Study the drawing (mm; zero at the part's minimum x, y, z) and answer. A direction names the side the tool comes from. Coordinates: 2 decimals unless noted, no trailing zeros. Write each loop counter-clockwise with the first axis right and the second up, starting at its lowest first coordinate (ties: lowest second). Pieces come first, ordered by that corner, then holes. Notation, with made-up numbers: M 55.25,-1.75 L 108.25,-1.75 A25 ccw 108.25,11.25 Z; hole C 55.5,74.25 d11. An arc over 180 degrees is marked long. Answer as a JSON object with one key per item and string values. Group by question number.
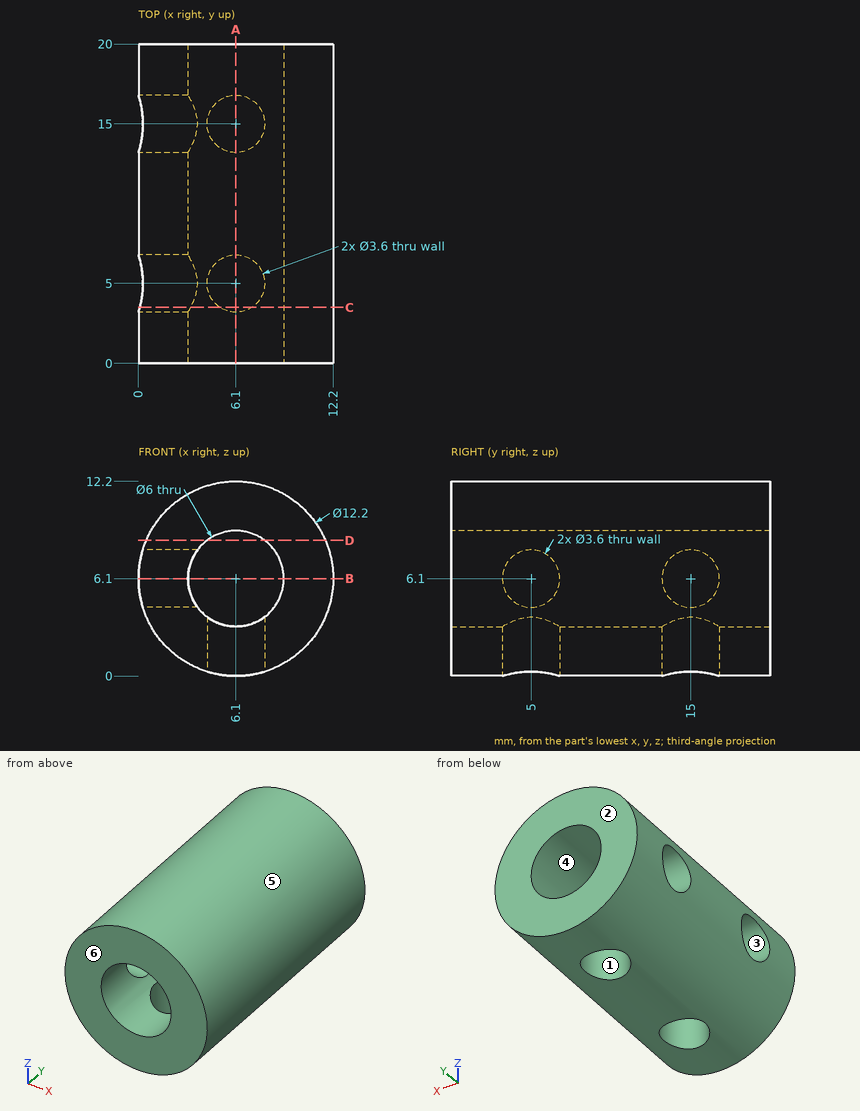
Item 1: A cutting plane is placed at B-B, the plane z = 6.1. Write down the section's boundary in (x, y).
Item 2: Consider L1, parallel to Y at x = 0.8, z = 6.1; L2, parallel to Y at x = 2.5, z = 5; L3, parallel to Z at x = 5, y = 11.5. Determine where each line is inside the solid, lowest interval first. Write a range as from..to.
Item 3: A cutting plane is placed at A-A, the plane x = 6.1. Write down the section's boundary in (y, z).
Item 4: Flat-ended cylindrical pins translate along their axes: pin 1 Ø3 at (x, y) = (6.1, 15) entering from -Z; pin 2 Ø1.5 at (y, z) = (14, 8.5) entering from -X; pin 3 Ø3 at (y, z) = (5, 6.1) entering from -X. Find the tip coordinate at first contact, or state that the pin passes through.
Item 5: A cutting plane is placed at D-D, the plane z = 8.5. Write down the section's boundary in (x, y).
Item 6: A cutting plane is placed at C-C, the plane y = 3.5. Write down the section's boundary in (x, z).
Item 7: For a pull along X with two mould halves and no side action, classify the marked faces 4, 5 and 6 as +X half, -X half, draft (parallel to the pull), parting line (faces both ways), or undercut.
Item 8: A tool of negligible diameter and unlimited length cuts with its end or side. For the marked faces 1, 2 and 3, from which of +Z, -Z, +X, -X, +Y, -Y can it reach the whole face along a straight path? Write none if from no direction.
Answer:
{
 "1": {"outline": "M 0,0 L 3.1,0 L 3.1,3.2 L 0,3.2 Z; M 0,6.8 L 3.1,6.8 L 3.1,13.2 L 0,13.2 Z; M 0,16.8 L 3.1,16.8 L 3.1,20 L 0,20 Z; M 9.1,0 L 12.2,0 L 12.2,20 L 9.1,20 Z"},
 "2": {"L1": "0..3.2, 6.8..13.2, 16.8..20", "L2": "0..3.58, 6.42..13.58, 16.42..20", "L3": "0.1..3.31, 8.89..12.1"},
 "3": {"outline": "M 0,0 L 3.2,0 L 3.2,3.1 L 0,3.1 Z; M 0,9.1 L 20,9.1 L 20,12.2 L 0,12.2 Z; M 6.8,0 L 13.2,0 L 13.2,3.1 L 6.8,3.1 Z; M 16.8,0 L 20,0 L 20,3.1 L 16.8,3.1 Z"},
 "4": {"pin 1": "z = 8.7", "pin 2": "x = 0.23", "pin 3": "x = 8.7"},
 "5": {"outline": "M 0.49,0 L 4.3,0 L 4.3,20 L 0.49,20 Z; M 7.9,0 L 11.71,0 L 11.71,20 L 7.9,20 Z"},
 "6": {"outline": "M 0.08,5.11 A6.1 ccw 5.11,0.08 L 5.11,3.27 A3 cw 3.27,5.11 Z; M 0.08,7.09 L 3.27,7.09 A3 cw long 7.09,3.27 L 7.09,0.08 A6.1 ccw long Z"},
 "7": {"face 4": "undercut", "face 5": "parting line", "face 6": "draft"},
 "8": {"face 1": "-Z", "face 2": "+Z, -Z, +X, -X, +Y", "face 3": "-X"}
}
